Here's how the part is built. I have some questions about the finished solid (model axes, mm). Face numbers are marked on the shaded views. Round coordinates to 2 decimals unless told otherwise and drop trailing zeros. Order: outer loops, then holes, each group sorted by start corner. A loop starts at its lowest first (then second) coordinate and runs counter-clockwise, first axis right, second up. Notation, with made-up numbers: (28.25, 80) -> (61.25, 80) arc R37 ccw to (61.25, 119) -> close; hole circle Ø6 at (3, -0.75). An arc over 180 degrees is marked (long way). Answer in a Markdown table with one row per item.
```python
from build123d import *

# Parameters (mm, degrees)
SKETCH_1_R          = 5
EXTRUDE_1_DEPTH     = 40
CUT_EXTRUDE_1_DEPTH = 7
SKETCH_4_R          = 6.5
SKETCH_4_R_2        = 2.5
CUT_EXTRUDE_4_DEPTH = 10
EXTRUDE_START       = -7
SKETCH_7_R          = 5
EXTRUDE_2_DEPTH     = 7
SKETCH_10_R         = 6.5
SKETCH_10_R_2       = 2.5
CUT_EXTRUDE_5_DEPTH = 5
FILLET_3_R          = 2
FILLET_4_R          = 2
FILLET_5_R          = 2


with BuildPart() as part:
    # Эскиз1 → Бобышка-Вытянуть1 (new body)
    with BuildSketch(Plane.XY):
        Circle(SKETCH_1_R)
    extrude(amount=EXTRUDE_1_DEPTH)

    # Эскиз3 → Вырез-Вытянуть1 (cut)
    with BuildSketch(Plane(origin=(0, 0, 0), x_dir=(-1, 0, 0), z_dir=(0, 0, -1))):
        with BuildLine():
            Line((-2.2, -2.323790008), (-2.2, 2.323790008))
            ThreePointArc((-2.2, 2.323790008), (0, 3.2), (2.2, 2.323790008))
            Line((2.2, 2.323790008), (2.2, -2.323790008))
            ThreePointArc((2.2, -2.323790008), (0, -3.2), (-2.2, -2.323790008))
        make_face()
    extrude(amount=-CUT_EXTRUDE_1_DEPTH, mode=Mode.SUBTRACT)

    # Эскиз4 → Вырез-Вытянуть-Тонкостенный4 (cut)
    with BuildSketch(Plane.XY.offset(40)):
        Circle(SKETCH_4_R)
        Circle(SKETCH_4_R_2, mode=Mode.SUBTRACT)
    extrude(amount=-CUT_EXTRUDE_4_DEPTH, mode=Mode.SUBTRACT)

    # Эскиз7 → Бобышка-Вытянуть2 (add)
    with BuildSketch(Plane.XY.offset(40).offset(EXTRUDE_START)):
        Circle(SKETCH_7_R)
    extrude(amount=EXTRUDE_2_DEPTH)

    # Эскиз10 → Вырез-Вытянуть-Тонкостенный5 (cut)
    with BuildSketch(Plane.XY.offset(40)):
        Circle(SKETCH_10_R)
        Circle(SKETCH_10_R_2, mode=Mode.SUBTRACT)
    extrude(amount=-CUT_EXTRUDE_5_DEPTH, mode=Mode.SUBTRACT)

    # Скругление3
    fillet_3_edges = [part.edges().sort_by_distance(p)[0] for p in [
        (-5, 0, 30),
    ]]
    fillet(fillet_3_edges, radius=FILLET_3_R)

    # Скругление4
    fillet_4_edges = [part.edges().sort_by_distance(p)[0] for p in [
        (-5, 0, 33),
    ]]
    fillet(fillet_4_edges, radius=FILLET_4_R - 0.0001)  # a hair under: the kernel refuses the full size

    # Скругление5
    fillet_5_edges = [part.edges().sort_by_distance(p)[0] for p in [
        (-2.5, 0, 30),
    ]]
    fillet(fillet_5_edges, radius=FILLET_5_R)

    # Скругление6: read off the stored shape, not the designer's step
    # Скругление6 outline → Скругление6 (revolve)
    with BuildSketch(Plane.XZ):
        with BuildLine():
            Line((3.726034838, 33.136435294), (3, 33.136435294))
            Line((3, 33.136435294), (3, 33))
            Line((3, 33), (2.5, 33))
            Line((2.5, 33), (2.5, 31.708099244))
            ThreePointArc((2.5, 31.708099244), (2.934473908, 32.575522915), (3.726034838, 33.136435294))
        make_face()
    revolve(axis=Axis((0, 0, 0), (0, 0, 1)))


solid = part.part
```
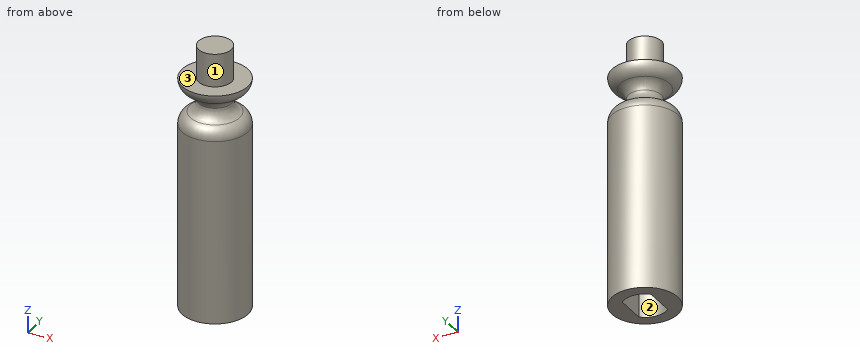
1. Suppose I cut it at A-A on z = 21. Write out the boundary of the cut face in (x, y).
Numbers:
| item | result |
|---|---|
| outline | circle Ø10 at (0, 0) |
2. Please list where these lines run through material, in increasing order: line 1 along Z through (x, y) = (-3.5, -0.5); line 2 along Z through (x, y) = (-1.5, 1); line 3 along Z through (x, y) = (1.25, 3).
Numbers:
| item | result |
|---|---|
| line 1 | z = 0 to 29.96, 33.05 to 35 |
| line 2 | z = 7 to 40 |
| line 3 | z = 0 to 30.15, 32.87 to 35 |
3. We'd pull the mould along Y, two halves only. Please class the marked faces 1, 2 and 3: released by +Y, released by -Y, zero draft, split by the parting line, or undercut.
Numbers:
| item | result |
|---|---|
| face 1 | split by the parting line |
| face 2 | undercut |
| face 3 | zero draft |
4. For pin 1 Ø1 at (x, y) = (-3, 1) entering from +Z; pin 2 Ø1.5 at (x, z) = (2, 33.5) entering from +Y; pin 3 Ø1.5 at (x, z) = (-2.5, 9.5) entering from +Y, each with a flat end and sliding along its axis, tell me the tip position at first contact or that it passes through.
Numbers:
| item | result |
|---|---|
| pin 1 | stops at z = 35 |
| pin 2 | stops at y = 4.53 |
| pin 3 | stops at y = 4.68 |
